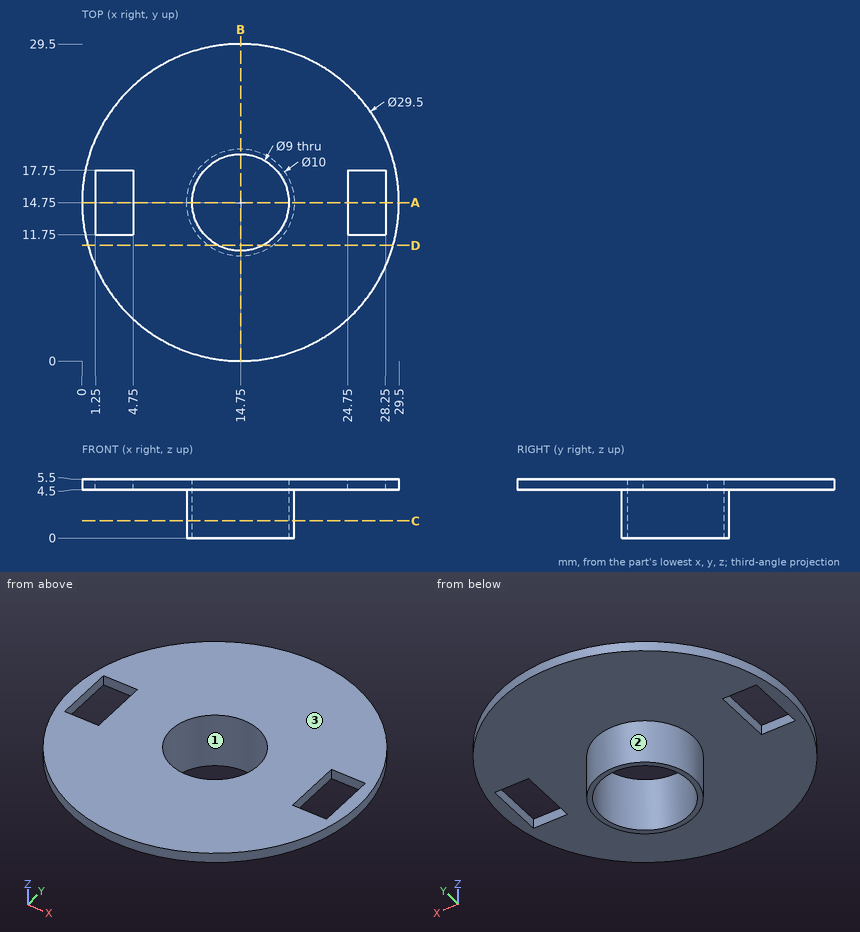
Verification items for this drawing (mm, ordinates from the low corner). Give positions to 0.01 mm unless a question says otherwise; leave off trailing zeros. Loops run counter-clockwise (first coordinate to the right, second up) from the corner with the lowest first, then second, coordinate; pieces in that order, holes last.
(1) Depth check by flat-ended pin: pin 1 Ø0.8 at (y, z) = (15, 5) entering from +X; pin 2 Ø1 at (x, z) = (15, 3.5) entering from +Y; pin 3 Ø0.8 at (y, z) = (13.5, 5) entering from -X; pin 4 Ø0.5 at (x, z) = (2.5, 5) entering from +Y. Enter the tip coordinate at first touch or a pass-through.
From the geometry:
pin 1: stops at x = 29.5
pin 2: stops at y = 19.75
pin 3: stops at x = 0.02
pin 4: stops at y = 23.33
(2) Thickness scan on L1, parallel to Y at x = 14.75, z = 3.8; L2, parallel to Z at x = 16.25, y = 22.25; L3, parallel to Y at x = 16.25, z = 5.1. Record the ranges inside material, lowest first.
From the geometry:
L1: y = 9.75 to 10.25, 19.25 to 19.75
L2: z = 4.5 to 5.5
L3: y = 0.08 to 10.51, 18.99 to 29.42
(3) Section check A-A on y = 14.75. Record the cut outline in (x, z).
From the geometry:
outline: (0, 4.5) - (1.25, 4.5) - (1.25, 5.5) - (0, 5.5) - close; (4.75, 4.5) - (9.75, 4.5) - (9.75, 0) - (10.25, 0) - (10.25, 5.5) - (4.75, 5.5) - close; (19.25, 0) - (19.75, 0) - (19.75, 4.5) - (24.75, 4.5) - (24.75, 5.5) - (19.25, 5.5) - close; (28.25, 4.5) - (29.5, 4.5) - (29.5, 5.5) - (28.25, 5.5) - close
(4) Section check B-B on x = 14.75. Record the cut outline in (y, z).
From the geometry:
outline: (0, 4.5) - (9.75, 4.5) - (9.75, 0) - (10.25, 0) - (10.25, 5.5) - (0, 5.5) - close; (19.25, 0) - (19.75, 0) - (19.75, 4.5) - (29.5, 4.5) - (29.5, 5.5) - (19.25, 5.5) - close
(5) Section check C-C on z = 1.6. Record the cut outline in (x, y).
From the geometry:
outline: circle Ø10 at (14.75, 14.75); hole circle Ø9 at (14.75, 14.75)
(6) Section check D-D on y = 10.75. Record the cut outline in (x, z), then the cut area to 3 significant figures.
From the geometry:
outline: (0.55, 4.5) - (11.75, 4.5) - (11.75, 0) - (12.69, 0) - (12.69, 5.5) - (0.55, 5.5) - close; (16.81, 0) - (17.75, 0) - (17.75, 4.5) - (28.95, 4.5) - (28.95, 5.5) - (16.81, 5.5) - close
area: 32.7 mm2
(7) Release check for a two-part mould opening along X. For the marked faces 1, 2 and 3 record: released by +X, released by -X, zero draft, split by the parting line, or undercut.
From the geometry:
face 1: undercut
face 2: split by the parting line
face 3: zero draft
